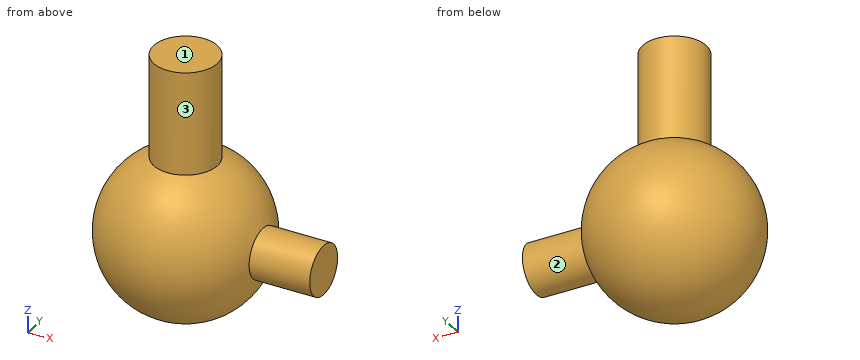
```python
from build123d import *

# Parameters (mm, degrees)
ESQUISSE2_R        = 2.5
BOSS_EXTRU_1_DEPTH = 14
ESQUISSE3_R        = 1.95
BOSS_EXTRU_2_DEPTH = 10


with BuildPart() as part:
    # Esquisse1 → Révolution3 (revolve)
    with BuildSketch(Plane.XY):
        with BuildLine():
            Line((0, 6.389898843), (0, -6.389898843))
            ThreePointArc((0, -6.389898843), (-6.389898843, 0), (0, 6.389898843))
        make_face()
    revolve(axis=Axis((0, 0, 0), (0, 1, 0)))

    # Esquisse2 → Boss.-Extru.1 (add)
    with BuildSketch(Plane.XY):
        with Locations(Location((0, 0, 0), (0, 0, 180))):
            Circle(ESQUISSE2_R)
    extrude(amount=BOSS_EXTRU_1_DEPTH)

    # Esquisse3 → Boss.-Extru.2 (add)
    with BuildSketch(Plane(origin=(0.84709995, 0, 0), x_dir=(0, 0, -1), z_dir=(1, 0, 0))):
        with Locations(Location((0, 0, 0), (0, 0, 180))):
            Circle(ESQUISSE3_R)
    extrude(amount=BOSS_EXTRU_2_DEPTH)


solid = part.part
```
Design review of the part built by this model. Coordinates are the model's own, in mm. Face numbers are marked on the shaded views. A direction names the side the tool comes from. Give positions to 0.01 mm unless a question says otherwise; leave off trailing zeros. Loops run counter-clockwise (first coordinate to the right, second up) from the corner with the lowest first, then second, coordinate; pieces in that order, holes last. Notation, with made-up numbers: M 63.25,6 L 93.25,6 A25 cw 93.25,32 Z; hole C 37,87.25 d6. An arc over 180 degrees is marked long. Return JSON: item names as keys, results as strings. Group by question number.
Item 1: For probe 1 along X at (y, z) = (-1.75, -2.5); probe 2 along X at (y, z) = (4.75, -3.5); probe 3 along Z at (x, y) = (4.75, 2), list the stretches that pass through material, from the lowest coordinate up.
Item 2: We need section A-A (y = 0). Give the boundary of the cut face in (x, z), and give its area (3 significant figures).
Item 3: Tool access review of the marked faces 1, 2 and 3: name each direction out of +Z, -Z, +X, -X, +Y, -Y from which nothing blocks a thin tool from reaching the whole face with its end or side.
Item 4: We need section D-D (x = 1.5). Give the boundary of the cut face in (y, z), and give its area (3 significant figures).
Item 5: We need section B-B (x = 9.5). Give the boundary of the cut face in (y, z), and give its area (3 significant figures).
Item 6: We need section C-C (z = 0). Give the boundary of the cut face in (x, y).
Item 7: Insertion check: pin 1 Ø5 at (x, y) = (-2, -5) entering from -Z; pin 2 Ø8 at (x, z) = (-1, 11.5) entering from -Y; pin 3 Ø2 at (y, z) = (3, 8) entering from +X; pin 4 Ø5 at (x, z) = (6, 7) entering from +Y. Each pin has a flat end and moves straight along its axis. Give the tip position at first contact, or say it passes through.
Output:
{
 "1": {"probe 1": "x = -5.61 to 5.61", "probe 2": "x = -2.45 to 2.45", "probe 3": "z = -3.78 to 3.78"},
 "2": {"outline": "M -2.5,5.88 A6.39 ccw long 6.09,-1.95 L 10.85,-1.95 L 10.85,1.95 L 6.09,1.95 A6.39 ccw 2.5,5.88 L 2.5,14 L -2.5,14 Z", "area": "185 mm^2"},
 "3": {"face 1": "+Z, +X, -X, +Y, -Y", "face 2": "+X", "face 3": "+Z"},
 "4": {"outline": "M -2,5.88 A6.21 ccw long 2,5.88 L 2,14 L -2,14 Z", "area": "153 mm^2"},
 "5": {"outline": "C 0,0 d3.9", "area": "11.9 mm^2"},
 "6": {"outline": "M 6.09,-1.95 L 10.85,-1.95 L 10.85,1.95 L 6.09,1.95 A6.39 ccw long Z"},
 "7": {"pin 1": "stops at z = -5.7", "pin 2": "stops at y = -2.5", "pin 3": "stops at x = 1.5", "pin 4": "passes through"}
}
